Could you check a few things on this model? Use its own coordinates, in mm. Face numbers are marked on the shaded views. A direction names the side the tool comes from. Give positions to 0.01 mm unless a question says otherwise; leave off trailing zeros. Loops run counter-clockwise (first coordinate to the right, second up) from the corner with the lowest first, then second, coordinate; pieces in that order, holes last. Notation, with made-up numbers: M 36,0.25 L 94,0.25 A19 ccw 94,5.25 Z; hole C 15,-6 d2. An arc over 180 degrees is marked long. Answer in a Markdown table with one row per item. Add a question column.
1. If we section it at D-D on z = -37: List the corners of the cut face in (x, y) for me, then the cut area to 3 significant figures.
2. If we section it at A-A on x = 5: List the corners of the cut face in (y, z) for me.
3. If we section it at B-B on z = -27: List the corners of the cut face in (x, y) for me.
4. If we section it at C-C on y = -10: List the corners of the cut face in (x, z) for me, then the cut area to 3 significant figures.
5. Which directions (+Z, -Z, +X, -X, +Y, -Y) give clear straight access to the entire face, cutting with the end or side of a thin tool? Please do the marked faces 4 and 5.
6. Thinking about a two-plate mould opening in Z: for the marked faces 1, 2 and 3, which applies, released by +Z, released by -Z, zero draft, split by the parting line, or undercut?
7. I'm going to push flat-ended pins straight in: pin 1 Ø5 at (y, z) = (0.5, -36) entering from +X; pin 2 Ø3 at (y, z) = (0, -18) entering from +X; pin 3 Ø5 at (x, y) = (25, 7.454) entering from -Z. Where does each tip first touch, or does it pass through?
8. I need wall thicknesses on line 1 along Y through (x, z) = (-3.5, -27); line 2 along Z through (x, y) = (4, 4.5); line 3 along Y through (x, z) = (24, -55) (3 decimals). Which ranges of each line are inside material? Lowest first, please. Write a range as from..to.
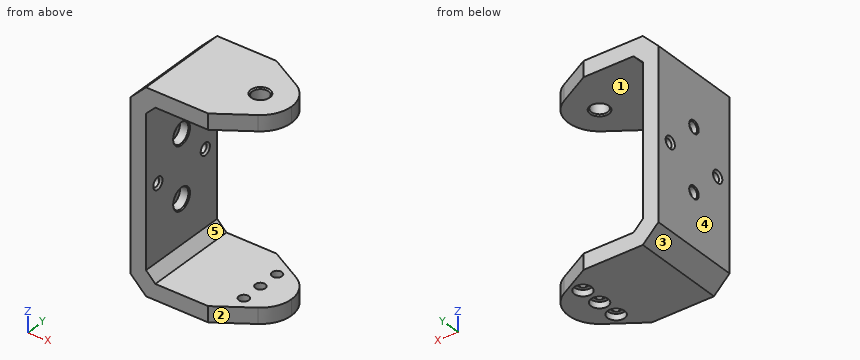
Solid Edge part; units mm, degrees
sketch "Sketch1" plane through (0, 0, 0) normal (0, -1, 0) x (1, 0, 0)
  line L0 (0, 0) -> (35, 0)
  line L1 (35, 0) -> (35, 5)
  line L2 (35, 5) -> (-5, 5)
  line L3 (-5, 5) -> (-5, -59)
  line L4 (-5, -59) -> (35, -59)
  line L5 (35, -59) -> (35, -54)
  line L6 (35, -54) -> (0, -54)
  line L7 (0, -54) -> (0, 0)
  dimension "D1" = 35
  dimension "D2" = 35
  dimension "D3" = 35
extrude "Protrusion1" add sketch "Sketch1" along normal mid plane 30
sketch "Sketch2" plane through (7.5, 0, 5) normal (0, 0, 1) x (0, 1, 0)
  line L0 (-15, -12.5) -> (-4.8551, -27.5)
  line L1 (-4.8551, -27.5) -> (6.4359, -27.5)
  line L2 (6.4359, -27.5) -> (15, -11.5446)
  line L3 (15, -11.5446) -> (15, -30)
  line L4 (15, -30) -> (-15, -30)
  line L5 (-15, -30) -> (-15, -12.5)
  dimension "D1" = 15
extrude "Cutout1" cut sketch "Sketch2" against normal through all
fillet "tip_round" radius 10 4 edges at (35, -4.8551, 2.5) (35, 6.4359, 2.5) (35, -4.8551, -56.5) (35, 6.4359, -56.5)
hole "bearing_hole" at (25, 0.454, 5) direction (0, 0, -1) diameter 5.3 end up to next start chamfer 0.4 start chamfer angle 45 end chamfer 0.4 end chamfer angle 45
hole "Hole_6" at (0, 0, -37) direction (-1, 0, 0) diameter 3.4 depth 30 tip angle 118 counterbore diameter 6.5 counterbore depth 3 start chamfer 0.3 start chamfer angle 45 end chamfer 0.3 end chamfer angle 45
hole "Hole1" at (0, 0, -17) direction (-1, 0, 0) diameter 3.4 depth 30 tip angle 118 counterbore diameter 6.5 counterbore depth 3 start chamfer 0.3 start chamfer angle 45 end chamfer 0.3 end chamfer angle 45
hole "Hole2" at (0, -10, -27) direction (-1, 0, 0) diameter 2.7 depth 30 tip angle 118 start chamfer 0.6 start chamfer angle 45 end chamfer 0.6 end chamfer angle 45
hole "Hole3" at (0, 10, -27) direction (-1, 0, 0) diameter 2.7 depth 30 tip angle 118 start chamfer 0.6 start chamfer angle 45 end chamfer 0.6 end chamfer angle 45
chamfer "core_chamfers" distance 3 angle 45 2 edges at (0, 0, 0) (0, 0, -54)
chamfer "outter_chamfers" distance 5 angle 45 2 edges at (-5, 0, 5) (-5, 0, -59)
hole "Hole4" at (25, 0.454, -59) direction (0, 0, 1) diameter 3.2 end up to next counterbore diameter 5.5 counterbore depth 2
hole "Hole5" at (25, -6.546, -59) direction (0, 0, 1) diameter 3.2 end up to next counterbore diameter 5.5 counterbore depth 2
hole "Hole6" at (25, 7.454, -59) direction (0, 0, 1) diameter 3.2 end up to next counterbore diameter 5.5 counterbore depth 2
properties material "Polypropylene, general purpose"
Results:
| question | item | result |
|---|---|---|
| 1 | outline | M -5,-15 L 0,-15 L 0,-3.55 L -0.3,-3.25 L -3,-3.25 L -3,-1.7 L -4.7,-1.7 L -5,-2 Z; M -5,2 L -4.7,1.7 L -3,1.7 L -3,3.25 L -0.3,3.25 L 0,3.55 L 0,15 L -5,15 Z |
| 1 | area | 124 mm2 |
| 2 | outline | M -15,-59 L 15,-59 L 15,-54 L -15,-54 Z; M -15,0 L 15,0 L 15,5 L -15,5 Z |
| 3 | outline | M -5,-15 L 0,-15 L 0,-11.95 L -0.6,-11.35 L -4.4,-11.35 L -5,-11.95 Z; M -5,-8.05 L -4.4,-8.65 L -0.6,-8.65 L 0,-8.05 L 0,8.05 L -0.6,8.65 L -4.4,8.65 L -5,8.05 Z; M -5,11.95 L -4.4,11.35 L -0.6,11.35 L 0,11.95 L 0,15 L -5,15 Z |
| 4 | outline | M -5,-54 L 0,-59 L 27.39,-59 L 27.39,-54 L 3,-54 L 0,-51 L 0,-28.95 L -0.6,-28.35 L -4.4,-28.35 L -5,-28.95 Z; M -5,-25.05 L -4.4,-25.65 L -0.6,-25.65 L 0,-25.05 L 0,-3 L 3,0 L 27.39,0 L 27.39,5 L 0,5 L -5,0 Z |
| 4 | area | 564 mm2 |
| 5 | face 4 | +Z, -Z, -X, +Y, -Y |
| 5 | face 5 | +X, +Y, -Y |
| 6 | face 1 | undercut |
| 6 | face 2 | zero draft |
| 6 | face 3 | released by -Z |
| 7 | pin 1 | x = 0 |
| 7 | pin 2 | x = -3 |
| 7 | pin 3 | z = -57 |
| 8 | line 1 | -15..-11.35, -8.65..8.65, 11.35..15 |
| 8 | line 2 | -59..-54, 0..5 |
| 8 | line 3 | -12.295..-7.795, -5.297..-0.795, 1.703..6.205, 8.703..12.34 |
